Verification items for the finished model (mm, model axes). Give positions to 0.01 mm unless a question says otherwise; leave off trailing zeros. Write each loop counter-clockwise with the first axis right and the second up, starting at its lowest first coordinate (ties: lowest second). Pieces come first, ordered by that corner, then holes.
from build123d import *

# Parameters (mm, degrees)
SKETCH1_R           = 34.925
BOSS_EXTRUDE1_DEPTH = 4.7625


with BuildPart() as part:
    # Sketch1 → Boss-Extrude1 (new body)
    with BuildSketch(Plane.XY):
        Circle(SKETCH1_R)
        with BuildLine():
            ThreePointArc((2.243888697, 8.727933453), (-0.797066547, 7.281111303), (-2.243888697, 10.322066547))
            ThreePointArc((-2.243888697, 10.322066547), (9.70011878, 20.108105734), (23.923949148, 14.099068603))
            ThreePointArc((23.923949148, 14.099068603), (23.396113859, 10.773096108), (20.070141364, 11.300931397))
            ThreePointArc((20.070141364, 11.300931397), (10.380475923, 15.394453179), (2.243888697, 8.727933453))
        make_face(mode=Mode.SUBTRACT)
        with BuildLine():
            ThreePointArc((2.243888697, -10.322066547), (-9.70011878, -20.108105734), (-23.923949148, -14.099068603))
            ThreePointArc((-23.923949148, -14.099068603), (-23.396113859, -10.773096108), (-20.070141364, -11.300931397))
            ThreePointArc((-20.070141364, -11.300931397), (-10.380475923, -15.394453179), (-2.243888697, -8.727933453))
            ThreePointArc((-2.243888697, -8.727933453), (0.797066547, -7.281111303), (2.243888697, -10.322066547))
        make_face(mode=Mode.SUBTRACT)
        with BuildLine():
            ThreePointArc((-5.712134337, -8.885472165), (-21.077597689, -7.359558154), (-26.886333692, 6.947239658))
            ThreePointArc((-26.886333692, 6.947239658), (-24.161280075, 8.92582145), (-22.182698283, 6.200767833))
            ThreePointArc((-22.182698283, 6.200767833), (-18.225627153, -3.545417318), (-7.758249844, -4.584912017))
            ThreePointArc((-7.758249844, -4.584912017), (-4.584912017, -5.712134337), (-5.712134337, -8.885472165))
        make_face(mode=Mode.SUBTRACT)
        with BuildLine():
            ThreePointArc((-10.322066547, -2.243888697), (-20.108105734, 9.70011878), (-14.099068603, 23.923949148))
            ThreePointArc((-14.099068603, 23.923949148), (-10.773096108, 23.396113859), (-11.300931397, 20.070141364))
            ThreePointArc((-11.300931397, 20.070141364), (-15.394453179, 10.380475923), (-8.727933453, 2.243888697))
            ThreePointArc((-8.727933453, 2.243888697), (-7.281111303, -0.797066547), (-10.322066547, -2.243888697))
        make_face(mode=Mode.SUBTRACT)
        with BuildLine():
            ThreePointArc((-8.885472165, 5.712134337), (-7.359558154, 21.077597689), (6.947239658, 26.886333692))
            ThreePointArc((6.947239658, 26.886333692), (8.92582145, 24.161280075), (6.200767833, 22.182698283))
            ThreePointArc((6.200767833, 22.182698283), (-3.545417318, 18.225627153), (-4.584912017, 7.758249844))
            ThreePointArc((-4.584912017, 7.758249844), (-5.712134337, 4.584912017), (-8.885472165, 5.712134337))
        make_face(mode=Mode.SUBTRACT)
        with BuildLine():
            ThreePointArc((6.201017431, 4.414629875), (4.414629875, 7.269366751), (7.269366751, 9.055754306))
            ThreePointArc((7.269366751, 9.055754306), (15.894637853, 4.263683482), (20.641911756, -4.386324314))
            ThreePointArc((20.641911756, -4.386324314), (18.840742957, -7.231758214), (15.995309056, -5.430589416))
            ThreePointArc((15.995309056, -5.430589416), (12.518320569, 0.90483132), (6.201017431, 4.414629875))
        make_face(mode=Mode.SUBTRACT)
    extrude(amount=BOSS_EXTRUDE1_DEPTH)


solid = part.part
Item 1: Sectioned sample at A-A on y = 12.7. Record the cut outline in (x, z).
Answer key:
outline: (-32.53, 0) - (-20.24, 0) - (-20.24, 4.76) - (-32.53, 4.76) - close; (-15.46, 0) - (-10.32, 0) - (-10.32, 4.76) - (-15.46, 4.76) - close; (-5.56, 0) - (-1.16, 0) - (-1.16, 4.76) - (-5.56, 4.76) - close; (4.82, 0) - (18.84, 0) - (18.84, 4.76) - (4.82, 4.76) - close; (24.38, 0) - (32.53, 0) - (32.53, 4.76) - (24.38, 4.76) - close
Item 2: Sectioned sample at C-C on y = -13. Record the cut outline in (x, z), then the cut area to 3 significant figures.
Answer key:
outline: (-32.42, 0) - (-24.36, 0) - (-24.36, 4.76) - (-32.42, 4.76) - close; (-18.51, 0) - (-5.15, 0) - (-5.15, 4.76) - (-18.51, 4.76) - close; (0.98, 0) - (32.42, 0) - (32.42, 4.76) - (0.98, 4.76) - close
area: 252 mm2
Item 3: Depth check by flat-ended pin: pin 1 (2 mm diameter, centred on x = 26.5, z = 4, fed in from -Y); pin 2 (1 mm diameter, centred on x = -16.5, y = 18, fed in from -Z). Enter the tip coordinate at first touch or a pass-through.
Answer key:
pin 1: stops at y = -23.86
pin 2: passes through
Item 4: Sectioned sample at B-B on x = 19. Record the cut outline in (y, z).
Answer key:
outline: (-29.3, 0) - (-7.19, 0) - (-7.19, 4.76) - (-29.3, 4.76) - close; (0.05, 0) - (12.55, 0) - (12.55, 4.76) - (0.05, 4.76) - close; (18.43, 0) - (29.3, 0) - (29.3, 4.76) - (18.43, 4.76) - close
Item 5: Scan lines: line 1 along Y through (x, z) = (13.5, 2.1); line 2 along Y through (x, z) = (10, 1.05); line 3 along X through (y, z) = (8, 3.8). Record each from-to range of solid material in increasing order.
Answer key:
line 1: y = -32.21 to -0.2, 6.28 to 15.36, 20.17 to 32.21
line 2: y = -33.46 to 2.88, 8.19 to 15.33, 20.15 to 33.46
line 3: x = -34 to -26.44, -22.63 to -19.76, -14.75 to -9.75, -4.7 to -1.83, 1.83 to 4.72, 10.45 to 34
